For this review, take the finished solid that the model builds, in its own axes (mm). Face numbers are marked on the shaded views. Coordinates: 2 decimals unless noted, no trailing zeros. One line per item, written item: value. Start each with the question number.
1) For probe 1 along Y at (x, z) = (133.5, -17.5); probe 2 along X at (y, z) = (25, -38); probe 3 along X at (y, z) = (-0.5, -18), list the stretches that pass through material, from the lowest coordinate up. Write a range as from..to.
2) For pin 1 Ø12 at (x, z) = (2, -25.5) entering from -Y; pin 2 Ø10 at (y, z) = (-62.5, -50) entering from -X; pin 3 Ø8 at (x, y) = (-17.5, -23.5) entering from -Z, all flat-tipped, find the tip position at first contact; note any pin that passes through.
3) Mouldability with a two-part tool opening along Y and no side actions: class the marked faces 1, 2 and 3 as released by +Y, released by -Y, zero draft, split by the parting line, or undercut.
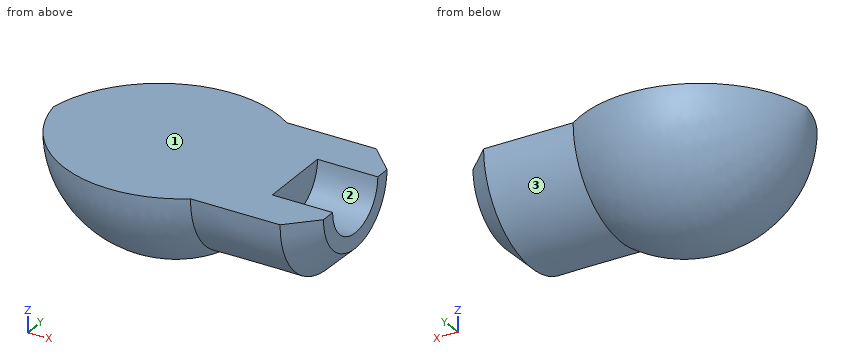
from build123d import *

# Parameters (mm, degrees)
REVOLVE1_ANGLE = 180


with BuildPart() as part:
    # Sketch2 → Revolve1 (revolve)
    with BuildSketch(Plane.XY):
        with BuildLine():
            Line((89.566728342, 37.93112192), (149.566728342, 37.93112192))
            Line((149.566728342, 37.93112192), (149.566728342, 52.93112192))
            Line((149.566728342, 52.93112192), (122.696670657, 79.801179605))
            Line((122.696670657, 79.801179605), (33.716670657, 79.801179605))
            ThreePointArc((33.716670657, 79.801179605), (-80.181557206, 91.138612278), (-150.433219191, 0.772425691))
            Line((-150.433219191, 0.772425691), (89.566728342, 0.93112192))
            Line((89.566728342, 0.93112192), (89.566728342, 37.93112192))
        make_face()
    revolve(axis=Axis((89.566728342, 0.93112192, 0), (-0.9999997813845841, -0.0006612342883058576, 0)), revolution_arc=REVOLVE1_ANGLE)


solid = part.part
Numbers:
1. probe 1: -64.88..-31.61, 33.53..66.71
1. probe 2: -133.4..149.58
1. probe 3: -146.11..89.58
2. pin 1: y = -92.45
2. pin 2: x = -105.21
2. pin 3: z = -96.82
3. face 1: zero draft
3. face 2: undercut
3. face 3: split by the parting line
